Part print with two shaded views. Sizes in mm from the minimum x, y, z corner. A direction names the side the tool comes from. Round coordinates to 2 decimals unless told otherwise and drop trailing zeros. Loops run counter-clockwise (first coordinate to the right, second up) from the corner with the lowest first, then second, coordinate; pieces in that order, holes last. Notation, with made-up numbers: M 30.5,37.5 L 84.5,37.5 A6 cw 84.5,42.5 Z; hole C 21,39 d3. An arc over 180 degrees is marked long. Answer as CSV lines item,"result". Start each with the question number.
Item 1: Band-saw the part on C-C (y = 4.7). Give the cut face in (x, z).
Item 2: Wall check: line 1 (Z direction, x = 10.75, y = 5); line 2 (X direction, y = 3.1, z = 4.5); line 3 (X direction, y = 3.5, z = 2.75). Give the ranges that are in metal, low to high.
Item 3: Mould opens along X. For the marked faces 3, 4 and 5 say: pulls with the +X half, pulls with the -X half, needs draft (parallel to the pull), parting line crosses it, or undercut.
Item 4: Band-saw the part on B-B (x = 6). Give the cut face in (y, z).
Item 5: Which spindle directions (+Z, -Z, +X, -X, +Y, -Y) get a long thin tool onto all of the face, cutting with end or side? Do the marked faces 1 and 2. Say none if no direction does.
Item 6: Band-saw the part on A-A (z = 5.5). Give the cut face in (x, y).
Item 7: Drop flat-ended pins along their axis: pin 1 Ø1.5 at (x, y) = (5, 5) entering from +Z; pin 2 Ø1.5 at (y, z) = (4, 3.5) entering from -X. Give the stop position or say it passes through.
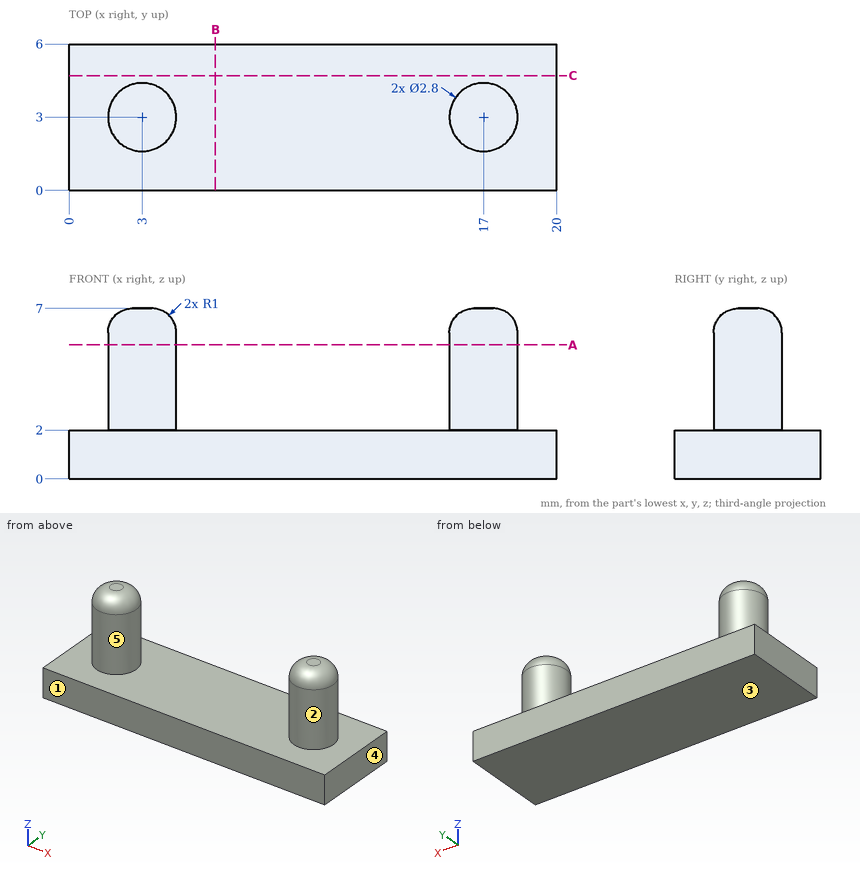
Answer block:
1,outline,"M 0,0 L 20,0 L 20,2 L 0,2 Z"
2,line 1,"z = 0 to 2"
2,line 2,"x = 1.6 to 4.4, 15.6 to 18.4"
2,line 3,"x = 1.69 to 4.31, 15.69 to 18.31"
3,face 3,"needs draft"
3,face 4,"pulls with the +X half"
3,face 5,"undercut"
4,outline,"M 0,0 L 6,0 L 6,2 L 0,2 Z"
5,face 1,"+Z, -Z, +X, -X, -Y"
5,face 2,"+Z"
6,outline,"C 3,3 d2.8; C 17,3 d2.8"
7,pin 1,"stops at z = 2"
7,pin 2,"stops at x = 1.62"
